The model under review builds one solid part; all positions refer to its coordinate system, in mm. Round coordinates to 2 decimals unless told otherwise and drop trailing zeros. Loops run counter-clockwise (first coordinate to the right, second up) from the corner with the lowest first, then second, coordinate; pieces in that order, holes last. Notation, with made-up numbers: (-22.75, 13.25) - (3.25, 13.25) arc R25 ccw to (3.25, 46.25) - close; hole circle Ø11 at (10, 41.25). An arc over 180 degrees is marked (long way). Answer as CSV lines item,"result".
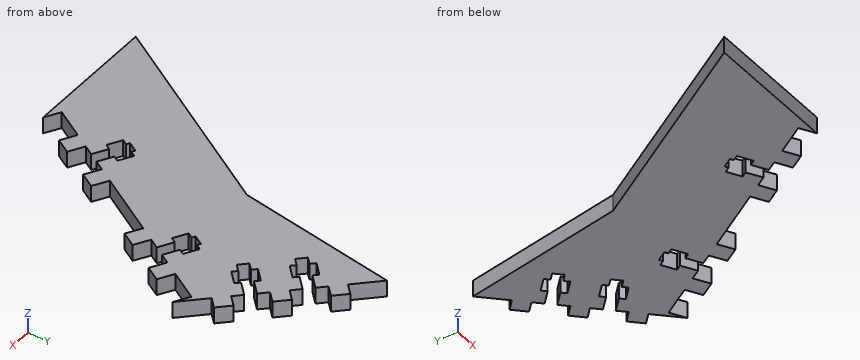
from build123d import *

# Parameters (mm, degrees)
BOSS_EXTRUDE1_DEPTH = 6.604
MOVE_FACE2_BY       = 0.00254
CUT_EXTRUDE1_DEPTH  = 374.058010856
CUT_EXTRUDE2_DEPTH  = 257.166060573
CUT_EXTRUDE3_DEPTH  = 257.166060573
BOSS_EXTRUDE2_DEPTH = 6.604


with BuildPart() as part:
    # Sketch1 → Boss-Extrude1 (new body)
    with BuildSketch(Plane.XY):
        Polygon((0, 304.426146906), (215.526146906, 88.9), (164.199707975, 0), (0, 0), (-164.199707975, 0), (-215.526146906, 88.9), align=None)
    extrude(amount=BOSS_EXTRUDE1_DEPTH)

    # Move Face2: a face moved outward by 0.00254
    extrude(part.faces().sort_by_distance((107.763073453, 196.663073453, 3.302))[0], amount=MOVE_FACE2_BY, dir=(0.707106781, 0.707106781, 0))

    # Sketch2 → Cut-Extrude1 (cut, through all)
    with BuildSketch(Plane.XY.offset(6.604)):
        Polygon((113.399707975, 0), (157.393798487, 76.2), (166.136053041, 138.293685968), (0.001796051, 304.427942957), (-215.526146906, 88.9), (-164.199707975, 0), align=None)
    extrude(amount=-CUT_EXTRUDE1_DEPTH, mode=Mode.SUBTRACT)

    # Sketch3 → Cut-Extrude2 (cut, through all)
    with BuildSketch(Plane.XY.offset(6.604)):
        Polygon((158.480476208, 3.302), (209.806915139, 92.202), (215.526146906, 88.9), (164.199707975, 0), align=None)
    extrude(amount=-CUT_EXTRUDE2_DEPTH, mode=Mode.SUBTRACT)

    # Sketch5 → Cut-Extrude3 (cut, through all)
    with BuildSketch(Plane.XY.offset(6.604)):
        Polygon((182.623803279, 121.805935729), (178.133675218, 117.315807669), (176.517229116, 118.932253771), (172.314469252, 114.729493906), (173.930915354, 113.113047804), (171.667890811, 110.850023262), (174.613414819, 107.904499254), (176.876439361, 110.167523796), (178.492885463, 108.551077695), (182.695645328, 112.753837559), (181.079199226, 114.370283661), (185.569327287, 118.860411722), align=None)
        Polygon((194.549583408, 100.899899479), (199.039711468, 105.39002754), (196.09418746, 108.335551548), (191.6040594, 103.845423487), (189.987613298, 105.461869589), (185.784853433, 101.259109724), (187.401299535, 99.642663622), (185.138274993, 97.37963908), (188.083799, 94.434115072), (190.346823543, 96.697139615), (191.963269645, 95.080693513), (196.166029509, 99.283453378), align=None)
        Polygon((198.148315139, 72.008712455), (192.649053825, 75.183712455), (193.792053825, 77.163446528), (188.644745235, 80.135246528), (187.501745235, 78.155512455), (186.269910701, 78.866712455), (184.187110701, 75.259197033), (185.418945235, 74.547997033), (184.275945235, 72.56826296), (189.423253825, 69.59646296), (190.566253825, 71.576197033), (196.065515139, 68.401197033), align=None)
        Polygon((172.221876208, 27.102802967), (166.722614894, 30.277802967), (167.865614894, 32.25753704), (162.718306304, 35.22933704), (161.575306304, 33.249602967), (160.34347177, 33.960802967), (158.26067177, 30.353287545), (159.492506304, 29.642087545), (158.349506304, 27.662353472), (163.496814894, 24.690553472), (164.639814894, 26.670287545), (170.139076208, 23.495287545), align=None)
    extrude(amount=-CUT_EXTRUDE3_DEPTH, mode=Mode.SUBTRACT)

    # Sketch6 → Boss-Extrude2 (add)
    with BuildSketch(Plane.XY.offset(6.604)):
        Polygon((178.528806488, 132.725927173), (175.116309162, 129.313429847), (179.606437222, 124.823301786), (183.018934548, 128.235799112), align=None)
        Polygon((188.586693343, 115.843045665), (191.999190669, 119.255542991), (196.48931873, 114.76541493), (193.076821404, 111.352917604), align=None)
        Polygon((205.469574851, 105.785158809), (209.959702911, 101.295030749), (206.547205585, 97.882533423), (202.057077525, 102.372661483), align=None)
        Polygon((209.176146906, 77.901477372), (203.456915139, 81.203477372), (200.281915139, 75.704216058), (206.001146906, 72.402216058), align=None)
        Polygon((193.931915139, 64.70569343), (199.651146906, 61.40369343), (196.476146906, 55.904432116), (190.756915139, 59.206432116), align=None)
        Polygon((183.249707975, 32.995567884), (177.530476208, 36.297567884), (174.355476208, 30.79830657), (180.074707975, 27.49630657), align=None)
        Polygon((168.005476208, 19.799783942), (173.724707975, 16.497783942), (170.549707975, 10.998522628), (164.830476208, 14.300522628), align=None)
    extrude(amount=-BOSS_EXTRUDE2_DEPTH)


solid = part.part
1. Take a section at B-B (x = 140.5). State the section outline as (y, z) points, plus the area to 3 significant figures.
Numbers:
outline,"(0, 0) - (46.94, 0) - (46.94, 6.6) - (0, 6.6) - close"
area,"310 mm²"
2. Wall thickness on probe 1 along Y at (x, z) = (182.5, 3.75); probe 2 along Y at (x, z) = (178, 2); probe 3 along Y at (x, z) = (193, 1.25): over which ranges is each line inside the solid? List them lowest first.
Numbers:
probe 1,"y = 31.7 to 33.43, 44.91 to 112.56, 112.95 to 115.79, 121.68 to 121.93, 127.72 to 128.75"
probe 2,"y = 28.69 to 36.03, 37.11 to 109.04, 117.45 to 132.2"
probe 3,"y = 57.91 to 70.17, 74.98 to 75.79, 77.62 to 96.12, 105.24 to 118.25"
3. Take a section at A-A (y = 57.5). State the section outline as (x, z) points, plus the area to 3 significant figures.
Numbers:
outline,"(146.6, 0) - (189.77, 0) - (189.77, 6.6) - (146.6, 6.6) - close; (193.71, 0) - (197.4, 0) - (197.4, 6.6) - (193.71, 6.6) - close"
area,"309 mm²"
